from build123d import *

# Parameters (mm, degrees)
F1_DEPTH = 13.5
F2_DEPTH = 2
F3_R     = 3.74999
F4_DEPTH = 2
F5_R     = 3.74999


# Not quite as in the source:
# - a fillet or chamfer is up to 0.001 mm smaller than in the source, because OpenCascade refuses the exact size
# - a feature names something its author has since deleted; it is built from what else it names


with BuildPart() as f1:
    # F0 (on Front) → F1 (new body)
    with BuildSketch(Plane.XZ):
        Polygon((2.2300408515, 13), (-27.2699591485, 13), (-27.2699591485, 10.2540537994), (-27.2699591485, 2.7540537994), (-27.2699591485, 0), (2.2300408515, 0), (2.2300408515, 2.75), (2.2300408515, 10.25), align=None)
    extrude(amount=F1_DEPTH)

    # F0 (on Front) → F2 (join)
    with BuildSketch(Plane.XZ):
        with BuildLine():
            Line((-27.2699591485, 2.7540537994), (-27.2699591485, 10.2540537994))
            Line((-27.2699591485, 10.2540537994), (-31.0199591485, 10.2540537994))
            Line((-31.0199591485, 10.2540537994), (-31.0199591485, 8.1040537994))
            ThreePointArc((-31.0199591485, 8.1040537994), (-29.8885882986, 7.6354246493), (-29.4199591485, 6.5040537994))
            ThreePointArc((-29.4199591485, 6.5040537994), (-31.0199591485, 4.9040537994), (-32.6199591485, 6.5040537994))
            Line((-32.6199591485, 6.5040537994), (-34.7699591485, 6.5040537994))
            Line((-34.7699591485, 6.5040537994), (-34.7699591485, 2.7540537994))
            Line((-34.7699591485, 2.7540537994), (-27.2699591485, 2.7540537994))
        make_face()
        with BuildLine():
            Line((-31.0199591485, 8.1040537994), (-31.0199591485, 10.2540537994))
            Line((-31.0199591485, 10.2540537994), (-34.7699591485, 10.2540537994))
            Line((-34.7699591485, 10.2540537994), (-34.7699591485, 6.5040537994))
            Line((-34.7699591485, 6.5040537994), (-32.6199591485, 6.5040537994))
            ThreePointArc((-32.6199591485, 6.5040537994), (-32.1513299984, 7.6354246493), (-31.0199591485, 8.1040537994))
        make_face()
    extrude(amount=F2_DEPTH)

    # F3 (radius 3.75 in the source; OpenCascade refuses exactly that, so slightly less here)
    f3_edges = [f1.edges().sort_by_distance(p)[0] for p in [
        (-34.769959, -1, 10.254054),
        (-34.769959, -1, 2.754054),
    ]]
    fillet(f3_edges, radius=F3_R)

    # F0 (on Front) → F4 (join)
    with BuildSketch(Plane.XZ):
        with BuildLine():
            Line((9.7300408515, 10.25), (2.2300408515, 10.25))
            Line((2.2300408515, 10.25), (2.2300408515, 2.75))
            Line((2.2300408515, 2.75), (5.9800408515, 2.75))
            Line((5.9800408515, 2.75), (5.9800408515, 4.9))
            ThreePointArc((5.9800408515, 4.9), (4.8486700016, 7.6313708499), (7.5800408515, 6.5))
            Line((7.5800408515, 6.5), (9.7300408515, 6.5))
            Line((9.7300408515, 6.5), (9.7300408515, 10.25))
        make_face()
        with BuildLine():
            Line((5.9800408515, 4.9), (5.9800408515, 2.75))
            Line((5.9800408515, 2.75), (9.7300408515, 2.75))
            Line((9.7300408515, 2.75), (9.7300408515, 6.5))
            Line((9.7300408515, 6.5), (7.5800408515, 6.5))
            ThreePointArc((7.5800408515, 6.5), (7.1114117014, 5.3686291501), (5.9800408515, 4.9))
        make_face()
    extrude(amount=F4_DEPTH)

    # F5 (radius 3.75 in the source; OpenCascade refuses exactly that, so slightly less here)
    f5_edges = [f1.edges().sort_by_distance(p)[0] for p in [
        (9.730041, -1, 10.25),
        (9.730041, -1, 2.75),
    ]]
    fillet(f5_edges, radius=F5_R)


solid = f1.part
Check sheet for the modelled part. Datum: model origin and axes. Units: mm. A direction names the side the tool comes from. Give positions to 0.01 mm unless a question says otherwise; leave off trailing zeros. Write each loop counter-clockwise with the first axis right and the second up, starting at its lowest first coordinate (ties: lowest second). Pieces come first, ordered by that corner, then holes. Notation, with made-up numbers: (49.5, 43.5) -> (70.5, 43.5) arc R16 cw to (70.5, 58.5) -> close; hole circle Ø2 at (-12.75, 87.5). An arc over 180 degrees is marked (long way). One line per item, written item: value. Start each with the question number.
Item 1: Gauge pin test, flat ends, axial feed: pin 1 (3.5 mm diameter, centred on x = 5.98, z = 6.5, fed in from +Y); pin 2 (4 mm diameter, centred on x = 6, z = 5.5, fed in from -Y); pin 3 (1 mm diameter, centred on y = -7, z = 4.5, fed in from +X); pin 4 (2 mm diameter, centred on x = 4.5, y = -1.5, fed in from +Z). Record the tip position at first contact, or that the pin passes through.
Item 2: Section check C-C on y = -5.5. Record the cut outline in (x, z).
Item 3: Section check B-B on x = -30.5. Record the cut outline in (y, z), then the cut area to 3 significant figures.
Item 4: Section check A-A on z = 6. Record the cut outline in (x, y), then the cut area to 3 significant figures.
Item 5: Tool access check on faces 1 (the flat face through (4, -1, 2.75)), 2 (the flat face through (4, -1, 10.25)), 3 (the flat face through (-29, -1, 10.254)). Record the directions out of +Z, -Z, +X, -X, +Y, -Y that give a thin tool (end or side, any length) a straight path to the whole face; none if there is none.
Item 6: Material ranges on probe 1 along X at (y, z) = (-0.8, 6.5); probe 2 along X at (y, z) = (-12.5, 7.75); probe 3 along Y at (x, z) = (3, 9), recorded low to high. Write a range as from..to.
Item 7: Section check D-D on z = 10.75. Record the cut outline in (x, y), then the cut area to 3 significant figures.
Results list:
1. pin 1: y = 0
1. pin 2: y = -2
1. pin 3: x = 2.23
1. pin 4: z = 10.25
2. outline: (-27.27, 0) -> (2.23, 0) -> (2.23, 13) -> (-27.27, 13) -> close
3. outline: (-2, 2.75) -> (0, 2.75) -> (0, 4.99) -> (-2, 4.99) -> close; (-2, 8.02) -> (0, 8.02) -> (0, 10.25) -> (-2, 10.25) -> close
3. area: 8.95 mm²
4. outline: (-34.74, -2) -> (-32.54, -2) -> (-32.54, 0) -> (-34.74, 0) -> close; (-29.5, -2) -> (-27.27, -2) -> (-27.27, -13.5) -> (2.23, -13.5) -> (2.23, -2) -> (4.46, -2) -> (4.46, 0) -> (-29.5, 0) -> close; (7.5, -2) -> (9.7, -2) -> (9.7, 0) -> (7.5, 0) -> close
4. area: 416 mm²
5. face 1: -Z, +X, +Y, -Y
5. face 2: +Z, +X, +Y, -Y
5. face 3: +Z, -X, +Y, -Y
6. probe 1: -34.77..-32.62, -29.42..4.38, 7.58..9.73
6. probe 2: -27.27..2.23
6. probe 3: -2..0
7. outline: (-27.27, -13.5) -> (2.23, -13.5) -> (2.23, 0) -> (-27.27, 0) -> close
7. area: 398 mm²
